Here's how the part is built. I have some questions about the finished solid (model axes, mm). A direction names the side the tool comes from. Round coordinates to 2 decimals unless told otherwise and drop trailing zeros. Write each loop counter-clockwise with the first axis right and the second up, starting at its lowest first coordinate (ties: lowest second). Pieces come first, ordered by that corner, then holes. Notation, with made-up numbers: (53.5, -9) -> (112.5, -9) arc R15 ccw to (112.5, 0) -> close; hole circle Ø4 at (81.25, 5.5). An arc over 180 degrees is marked (long way). Answer as CSV lines item,"result".
from build123d import *

# Parameters (mm, degrees)
SKETCH1_W           = 21.0312
SKETCH1_H           = 21.0312
BOSS_EXTRUDE1_DEPTH = 1.5875
SKETCH2_R           = 1.524
CUT_EXTRUDE1_DEPTH  = 15.9557963
FILLET1_R           = 2.54
SKETCH3_R           = 5.9817
BOSS_EXTRUDE2_DEPTH = 11.176
SKETCH4_R           = 6.35
BOSS_EXTRUDE3_DEPTH = 7.366
SKETCH5_R           = 3.8735
BOSS_EXTRUDE4_DEPTH = 4.064


with BuildPart() as part:
    # Sketch1 → Boss-Extrude1 (new body)
    with BuildSketch(Plane.XY):
        Rectangle(SKETCH1_W, SKETCH1_H)
    extrude(amount=BOSS_EXTRUDE1_DEPTH)

    # Sketch2 → Cut-Extrude1 (cut, through all)
    with BuildSketch(Plane.XY.offset(1.5875)):
        with Locations((-7.5438, 7.5438)):
            Circle(SKETCH2_R)
        with Locations((-7.5438, -7.5438)):
            Circle(SKETCH2_R)
        with Locations((7.5438, -7.5438)):
            Circle(SKETCH2_R)
        with Locations((7.5438, 7.5438)):
            Circle(SKETCH2_R)
    extrude(amount=-CUT_EXTRUDE1_DEPTH, mode=Mode.SUBTRACT)

    # Fillet1
    fillet1_edges = [part.edges().sort_by_distance(p)[0] for p in [
        (10.5156, -10.5156, 0.79375),
        (-10.5156, -10.5156, 0.79375),
        (-10.5156, 10.5156, 0.79375),
        (10.5156, 10.5156, 0.79375),
    ]]
    fillet(fillet1_edges, radius=FILLET1_R)

    # Sketch3 → Boss-Extrude2 (add)
    with BuildSketch(Plane.XY.offset(1.5875)):
        Circle(SKETCH3_R)
    extrude(amount=BOSS_EXTRUDE2_DEPTH)

    # Sketch4 → Boss-Extrude3 (add)
    with BuildSketch(Plane(origin=(0, 0, 0), x_dir=(-1, 0, 0), z_dir=(0, 0, -1))):
        with Locations(Location((0, 0, 0), (0, 0, 180))):
            Circle(SKETCH4_R)
    extrude(amount=BOSS_EXTRUDE3_DEPTH)

    # Sketch5 → Boss-Extrude4 (add)
    with BuildSketch(Plane(origin=(0, 0, -7.366), x_dir=(-1, 0, 0), z_dir=(0, 0, -1))):
        Circle(SKETCH5_R)
    extrude(amount=BOSS_EXTRUDE4_DEPTH)


solid = part.part
Item 1: Suppose I cut it at A-A, the plane x = 0. List the corners of the cut face in (y, z) for me.
Results found:
outline,"(-10.52, 0) -> (-6.35, 0) -> (-6.35, -7.37) -> (-3.87, -7.37) -> (-3.87, -11.43) -> (3.87, -11.43) -> (3.87, -7.37) -> (6.35, -7.37) -> (6.35, 0) -> (10.52, 0) -> (10.52, 1.59) -> (5.98, 1.59) -> (5.98, 12.76) -> (-5.98, 12.76) -> (-5.98, 1.59) -> (-10.52, 1.59) -> close"
Item 2: For faces 1 (the flat face through (5, -5, 1.588)), 2 (the cylindrical face through (6.02, -7.48, 0.8)), 3 (the flat face through (3, -3, -7.366)), which set-ups out of +Z, -Z, +X, -X, +Y, -Y let a thin tool reach every point of the face, with its end or its side?
Results found:
face 1,"+Z"
face 2,"+Z, -Z"
face 3,"-Z"
Item 3: Will these pins go through, and if not, where does the flat tip stop? pin 1 (6 mm diameter, centred on y = 0, z = -8, fed in from -X); pin 2 (6 mm diameter, centred on y = 5.5, z = -9, fed in from +X); pin 3 (3 mm diameter, centred on x = -4.5, z = 5.5, fed in from +Y) (3 decimals).
Results found:
pin 1,"stops at x = -6.35"
pin 2,"stops at x = 5.61"
pin 3,"stops at y = 5.175"
Item 4: If we mould it in two halves opening along X, with no side actions, what happens to faces 4 (the cylindrical face through (9.752, -9.791, 0.805)), 5 (the cylindrical face through (-9.791, 9.752, 0.805)), 6 (the cylindrical face through (-8, 9, 1))? For each: pulls with the +X half, pulls with the -X half, needs draft (parallel to the pull), parting line crosses it, or undercut.
Results found:
face 4,"pulls with the +X half"
face 5,"pulls with the -X half"
face 6,"undercut"
Item 5: Suppose I cut it at D-D, the plane z = -1. List the corners of the cut face in (x, y) for me.
Results found:
outline,"circle Ø12.7 at (0, 0)"
Item 6: Suppose I cut it at C-C, the plane z = 7.75. List the corners of the cut face in (x, y) for me, then the cut area to 3 significant figures.
Results found:
outline,"circle Ø11.96 at (0, 0)"
area,"112 mm²"
Item 7: I need wall thicknesses on L1, parallel to X at y = -8, z = 0.5; L2, parallel to Z at x = -1.5, y = -6.5; L3, parallel to Y at x = -0.25, z = -10. Which ranges of each line are inside material? Lowest first, please.
Results found:
L1,"x = -10.52 to -9, -6.09 to 6.09, 9 to 10.52"
L2,"z = 0 to 1.59"
L3,"y = -3.87 to 3.87"
